from build123d import *

# Parameters (mm, degrees)
F0_R     = 150
F1_DEPTH = 25
F2_R     = 21
F3_DEPTH = 160


with BuildPart() as f1:
    # F0 (on Top) → F1 (new body)
    with BuildSketch(Plane.XY):
        Circle(F0_R)
    extrude(amount=F1_DEPTH)

    # F2 (on face) → F3 (join)
    with BuildSketch(Plane.XY.offset(25)):
        Circle(F2_R)
    extrude(amount=F3_DEPTH)

    # F4 (on face) → F5 (revolve)
    with BuildSketch(Plane.XY.offset(185)):
        with BuildLine():
            Line((0, 21), (0, 40))
            ThreePointArc((0, 40), (-40, 0), (0, -40))
            Line((0, -40), (0, -21))
            ThreePointArc((0, -21), (-21, 0), (0, 21))
        make_face()
        with BuildLine():
            Line((0, -21), (0, 21))
            ThreePointArc((0, 21), (-21, 0), (0, -21))
        make_face()
    revolve(axis=Axis((0, 0, 185), (0, 1, 0)))


solid = f1.part
CAD build for the part. Positions are in the model's coordinates, mm. Coordinates: 2 decimals unless noted, no trailing zeros. Loops run counter-clockwise (first coordinate to the right, second up) from the corner with the lowest first, then second, coordinate; pieces in that order, holes last. Notation, with made-up numbers: (-36, -12.75) - (-22, -12.75) arc R21 ccw to (-22, -3.75) - close; hole circle Ø1 at (31, 13.25). An arc over 180 degrees is marked (long way). Write item = value, one per line. Start each with the question number.
Q1. Cut at D-D, the plane x = -126. List the corners of the cut face in (y, z), then the cut area to 3 significant figures.
Q2. Pull direction Z, two halves, no side cores. Call faces 1 (the cylindrical face through (-19.527, 148.724, 12.325)), 2 (the cylindrical face through (20.03, 6.31, 87.1)), 3 (the flat face through (-2, 2, 0)): pulls with the +Z half, pulls with the -Z half, needs draft (parallel to the pull), parting line crosses it, or undercut.
Q3. Drill centre lines: L1, parallel to Z at x = -38.5, y = -120; L2, parallel to Z at x = 32.5, y = -14; L3, parallel to Y at x = -28, z = 183.5. Where is each one in solid material? Low to high.
Q4. Flat gauge pins, fed straight in: pin 1 Ø1 at (x, y) = (-116, 97) entering from -Z; pin 2 Ø12 at (y, z) = (23.5, 113) entering from +X. Where does each tip first touch, or does it go through?
Q5. Cut at A-A, the plane x = 0. List the corners of the cut face in (y, z).
Q6. Cut at C-C, the plane z = 68.5. List the corners of the cut face in (x, y).
Computed:
q1.outline = (-81.39, 0) - (81.39, 0) - (81.39, 25) - (-81.39, 25) - close
q1.area = 4,070 mm²
q2.face_1 = needs draft
q2.face_2 = undercut
q2.face_3 = pulls with the -Z half
q3.L1 = 0 to 25
q3.L2 = 0 to 25, 166.35 to 203.65
q3.L3 = -28.53 to 28.53
q4.pin_1 = through
q4.pin_2 = 11.61
q5.outline = (-150, 0) - (150, 0) - (150, 25) - (21, 25) - (21, 150.96) arc R40 ccw (long way) to (-21, 150.96) - (-21, 25) - (-150, 25) - close
q6.outline = circle Ø42 at (0, 0)
